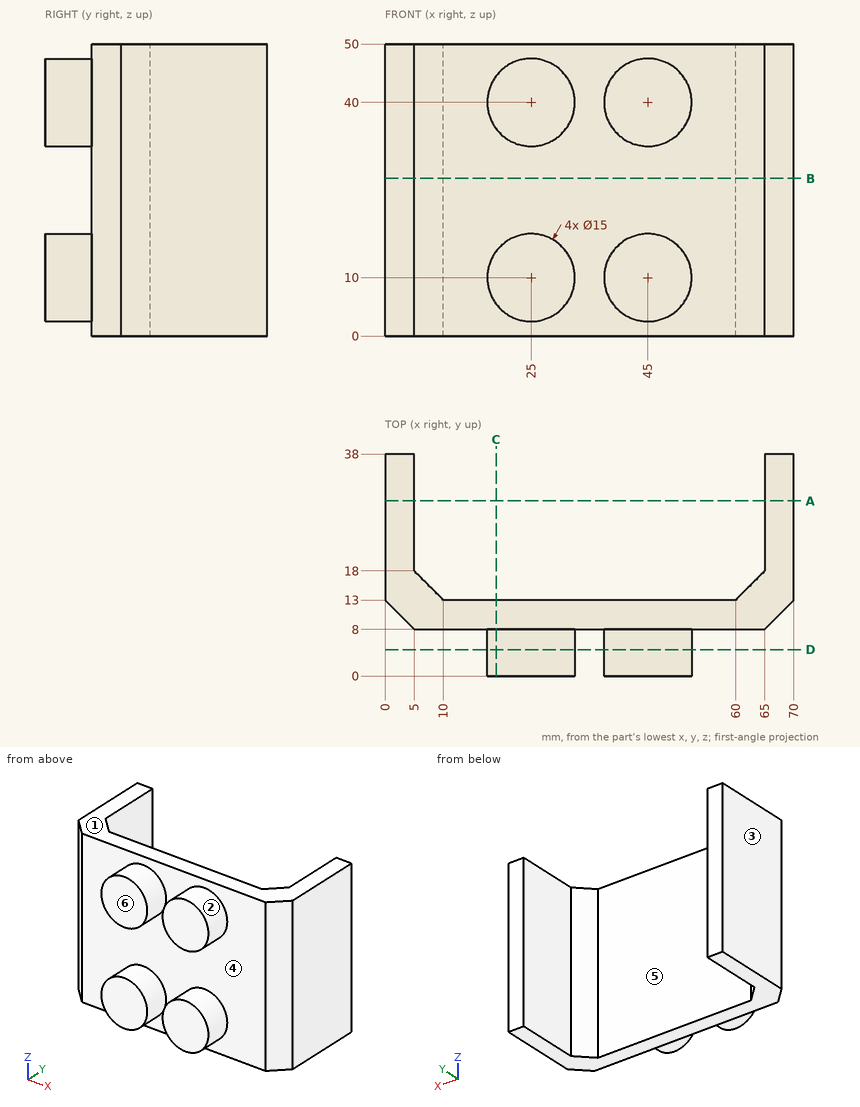
Study the drawing (mm; zero at the part's minimum x, y, z) and answer. A direction names the side the tool comes from. Round coordinates to 2 decimals unless told otherwise and drop trailing zeros. Order: outer loops, then holes, each group sorted by start corner. A loop starts at its lowest first (then second) coordinate and runs counter-clockwise, first axis right, second up. Notation, with made-up numbers: M 22,64.25 L 79,64.25 A15 cw 79,80.25 Z; hole C 82.5,59.5 d6. An arc over 180 degrees is marked long. One line per item, written item: value.
Q1. Straight lines are drawn through the part: line 1 (X direction, y = 33, z = 27); line 2 (Y direction, x = 60, z = 46.5); line 3 (Y direction, x = 20.5, z = 37). For each, find the intervals that lie inside material, in ascending order.
Derived:
line 1: 0 to 5, 65 to 70
line 2: 8 to 13
line 3: 0 to 13
Q2. Find section A-A on y = 30. Write down the section's boundary in (x, z).
Derived:
outline: M 0,0 L 5,0 L 5,50 L 0,50 Z; M 65,0 L 70,0 L 70,50 L 65,50 Z
Q3. Find section C-C on x = 19. Write down the section's boundary in (y, z), then the cut area to 3 significant figures.
Derived:
outline: M 0,5.5 L 8,5.5 L 8,0 L 13,0 L 13,50 L 8,50 L 8,44.5 L 0,44.5 L 0,35.5 L 8,35.5 L 8,14.5 L 0,14.5 Z
area: 394 mm²
Q4. Find section D-D on y = 4.5. Write down the section's boundary in (x, z).
Derived:
outline: C 25,10 d15; C 25,40 d15; C 45,10 d15; C 45,40 d15
Q5. Find section B-B on z = 27. Write down the section's boundary in (x, y), then the cut area to 3 significant figures.
Derived:
outline: M 0,13 L 5,8 L 65,8 L 70,13 L 70,38 L 65,38 L 65,18 L 60,13 L 10,13 L 5,18 L 5,38 L 0,38 Z
area: 600 mm²
Q6. A flat-ended cylindrical pin translates along its axis: pin 1 (8 mm diameter, centred on x = 38.5, z = 16.5, fed in from +Y). Find the tip coordinate at first contact, or state that the pin passes through.
Derived:
pin 1: y = 13
Q7. Determine the mould class of the marked faces 1, 2 and 3 for opening direction X: released by +X, released by -X, zero draft, split by the parting line, or undercut.
Derived:
face 1: zero draft
face 2: undercut
face 3: released by -X
Q8. For the marked faces 4, 5 and 6, determine the directions among +Z, -Z, +X, -X, +Y, -Y from which every point of the face is accessible in a straight line to the end or side of a thin tool.
Derived:
face 4: -Y
face 5: +Z, -Z, +Y
face 6: +Z, -Z, +X, -X, -Y
